from build123d import *

# Parameters (mm, degrees)
SKETCH1_R           = 2.0193
SKETCH1_W           = 41.91
SKETCH1_H           = 5.304051748
BOSS_EXTRUDE1_DEPTH = 3


with BuildPart() as part:
    # Sketch1 → Boss-Extrude1 (new body)
    # profile 1 of 2: a face of its own
    with BuildSketch(Plane(origin=(0, 0, 0), x_dir=(1, 0, 0), z_dir=(0, 1, 0))):
        Polygon((0.189585243, 26.171402615), (0.189585243, 20.867350867), (0.189585243, -0.722649133), (-41.720414757, -0.722649133), (-41.720414757, 8.08226518), (-41.720414757, 12.010049159), (-41.720414757, 20.867350867), (-41.720414757, 26.171402615), (-56.653469857, 26.171402615), (-56.653469857, -6.026700881), (8.402064139, -6.026700881), (8.402064139, 26.171402615), align=None)
        with Locations(Location((-44.895414757, 4.992350867, 0), (0, 0, 270))):
            Circle(SKETCH1_R, mode=Mode.SUBTRACT)
        with Locations(Location((3.364585243, 4.992350867, 0), (0, 0, 270))):
            Circle(SKETCH1_R, mode=Mode.SUBTRACT)
        with Locations(Location((-44.895414757, 15.152350867, 0), (0, 0, 270))):
            Circle(SKETCH1_R, mode=Mode.SUBTRACT)
        with Locations(Location((3.364585243, 15.152350867, 0), (0, 0, 270))):
            Circle(SKETCH1_R, mode=Mode.SUBTRACT)
    # profile 2 of 2: a face of its own
    with BuildSketch(Plane(origin=(0, 0, 0), x_dir=(1, 0, 0), z_dir=(0, 1, 0))):
        with Locations((-20.765414757, 23.519376741)):
            Rectangle(SKETCH1_W, SKETCH1_H)
    extrude(amount=BOSS_EXTRUDE1_DEPTH)


solid = part.part
Here's how the part is built. I have some questions about the finished solid (model axes, mm). A direction names the side the tool comes from. Coordinates: 2 decimals unless noted, no trailing zeros. Order: outer loops, then holes, each group sorted by start corner. A loop starts at its lowest first (then second) coordinate and runs counter-clockwise, first axis right, second up.
Item 1: If we section it at C-C on z = -5.5: List the corners of the cut face in (x, y) for me, plus the area to 3 significant figures.
Result sheet:
outline: (-56.65, 0) - (-46.85, 0) - (-46.85, 3) - (-56.65, 3) - close; (-42.94, 0) - (-41.72, 0) - (-41.72, 3) - (-42.94, 3) - close; (0.19, 0) - (1.41, 0) - (1.41, 3) - (0.19, 3) - close; (5.32, 0) - (8.4, 0) - (8.4, 3) - (5.32, 3) - close
area: 46.0 mm2
Item 2: If we section it at D-D on y = 2.5: List the corners of the cut face in (x, z) for me, plus the area to 3 significant figures.
Result sheet:
outline: (-56.65, -26.17) - (8.4, -26.17) - (8.4, 6.03) - (-56.65, 6.03) - close; hole circle Ø4.04 at (-44.9, -15.15); hole circle Ø4.04 at (-44.9, -4.99); hole (-41.72, -20.87) - (0.19, -20.87) - (0.19, 0.72) - (-41.72, 0.72) - close; hole circle Ø4.04 at (3.36, -15.15); hole circle Ø4.04 at (3.36, -4.99)
area: 1,140 mm2
Item 3: For P1, Ø3.5, axis at x = -44.9, z = -15.15, coming from the +Y side, with a flat end and sliding along its axis, tell me the tip position at first contact or that it passes through.
Result sheet:
P1: passes through
Item 4: If we section it at A-A on x = -46: List the corners of the cut face in (y, z) for me.
Result sheet:
outline: (0, -26.17) - (3, -26.17) - (3, -16.84) - (0, -16.84) - close; (0, -13.46) - (3, -13.46) - (3, -6.68) - (0, -6.68) - close; (0, -3.3) - (3, -3.3) - (3, 6.03) - (0, 6.03) - close
Item 5: If we mould it in two halves opening along Z, with no side actions, what happens to faces 1 (the face through (-25, 1, -26.171)), 2 (the face through (0.19, 1, -10)), 3 (the face through (-56.653, 1, -10))? For each: +Z half, -Z half, draft (parallel to the pull), parting line (faces both ways), or undercut.
Result sheet:
face 1: -Z half
face 2: undercut
face 3: draft
Item 6: For faces 4 (the face through (-21, 1, -20.867)), 5 (the face through (-25, 1, 6.027)), which set-ups out of +Z, -Z, +X, -X, +Y, -Y let a thin tool reach every point of the face, with its end or its side?
Result sheet:
face 4: +Y, -Y
face 5: +Z, +X, -X, +Y, -Y
Item 7: If we section it at B-B on z = 0: List the corners of the cut face in (x, y) for me, plus the area to 3 significant figures.
Result sheet:
outline: (-56.65, 0) - (-41.72, 0) - (-41.72, 3) - (-56.65, 3) - close; (0.19, 0) - (8.4, 0) - (8.4, 3) - (0.19, 3) - close
area: 69.4 mm2
Item 8: I need wall thicknesses on line 1 (Z direction, x = -31.5, y = 0.25); line 2 (X direction, y = 2.65, z = -10); line 3 (X direction, y = 2.55, z = -4.5). Which ranges of each line are inside material? Lowest first, please.
Result sheet:
line 1: z = -26.17 to -20.87, 0.72 to 6.03
line 2: x = -56.65 to -41.72, 0.19 to 8.4
line 3: x = -56.65 to -46.85, -42.94 to -41.72, 0.19 to 1.41, 5.32 to 8.4
